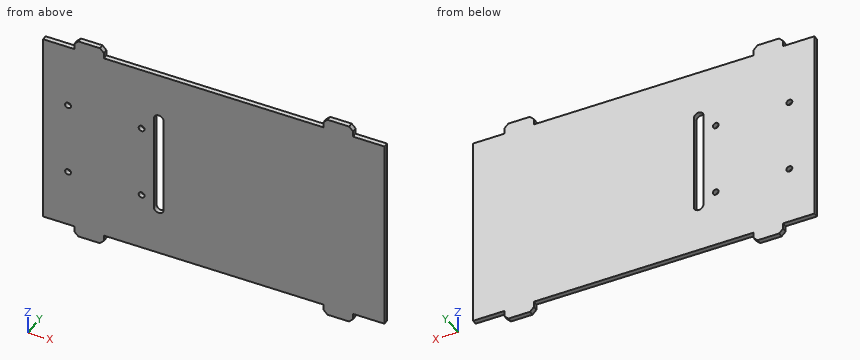
```python
from build123d import *

# Parameters (mm, degrees)
SKETCH1_W           = 174
SKETCH1_H           = 100
BOSS_EXTRUDE1_DEPTH = 2.5
SKETCH2_W           = 15
SKETCH2_H           = 2.5
BOSS_EXTRUDE2_DEPTH = 5
CHAMFER1_SIZE       = 2


with BuildPart() as part:
    # Sketch1 → Boss-Extrude1 (new body)
    with BuildSketch(Plane(origin=(0, 0, 0), x_dir=(1, 0, 0), z_dir=(0, 1, 0))):
        Rectangle(SKETCH1_W, SKETCH1_H)
        with BuildLine():
            Line((-25.5, 25), (-25.5, -25))
            ThreePointArc((-25.5, -25), (-28, -27.5), (-30.5, -25))
            Line((-30.5, -25), (-30.5, 25))
            ThreePointArc((-30.5, 25), (-28, 27.5), (-25.5, 25))
        make_face(mode=Mode.SUBTRACT)
        with BuildLine():
            ThreePointArc((-36.73295862, -15.609359563), (-38.23295862, -17.109359563), (-36.73295862, -18.609359563))
            ThreePointArc((-36.73295862, -18.609359563), (-35.23295862, -17.109359563), (-36.73295862, -15.609359563))
        make_face(mode=Mode.SUBTRACT)
        with BuildLine():
            ThreePointArc((-36.73295862, 18.890640437), (-35.23295862, 20.390640437), (-36.73295862, 21.890640437))
            ThreePointArc((-36.73295862, 21.890640437), (-38.23295862, 20.390640437), (-36.73295862, 18.890640437))
        make_face(mode=Mode.SUBTRACT)
        with BuildLine():
            ThreePointArc((-74.23295862, 21.890640437), (-75.73295862, 20.390640437), (-74.23295862, 18.890640437))
            ThreePointArc((-74.23295862, 18.890640437), (-72.73295862, 20.390640437), (-74.23295862, 21.890640437))
        make_face(mode=Mode.SUBTRACT)
        with BuildLine():
            ThreePointArc((-74.23295862, -15.609359563), (-75.73295862, -17.109359563), (-74.23295862, -18.609359563))
            ThreePointArc((-74.23295862, -18.609359563), (-72.73295862, -17.109359563), (-74.23295862, -15.609359563))
        make_face(mode=Mode.SUBTRACT)
    extrude(amount=BOSS_EXTRUDE1_DEPTH)

    # Sketch2 → Boss-Extrude2 (add)
    with BuildSketch(Plane.XY.offset(50)):
        with Locations((-63.5, 1.25)):
            Rectangle(SKETCH2_W, SKETCH2_H)
        with Locations((63.5, 1.25)):
            Rectangle(SKETCH2_W, SKETCH2_H)
    boss_extrude2 = extrude(amount=BOSS_EXTRUDE2_DEPTH)

    # Mirror1: Boss-Extrude2 across plane
    add(boss_extrude2.mirror(Plane.XY))

    # Chamfer1
    chamfer1_edges = [part.edges().sort_by_distance(p)[0] for p in [
        (-71, 1.25, 55),
        (-56, 1.25, 55),
        (56, 1.25, 55),
        (71, 1.25, 55),
        (-56, 1.25, -55),
        (-71, 1.25, -55),
        (71, 1.25, -55),
        (56, 1.25, -55),
    ]]
    chamfer(chamfer1_edges, length=CHAMFER1_SIZE)


solid = part.part
```
Source: CAD feature listing. Evaluate the final solid. Frame: model axes, mm. Round coordinates to 2 decimals unless told otherwise and drop trailing zeros. Loops run counter-clockwise (first coordinate to the right, second up) from the corner with the lowest first, then second, coordinate; pieces in that order, holes last. Notation, with made-up numbers: M -18.5,87 L -11.5,87 A8 ccw -11.5,95 Z; hole C -4.75,61 d9. An arc over 180 degrees is marked long. Use a Markdown table: item, result. Add a question column.
1. Cut plane C-C, the plane x = 17.5. Output: boundary loops of the cut face in (y, z), and give its area (3 significant figures).
2. Cut plane D-D, the plane y = 1.4. State how many separate pieces and enclosed holes the cut face has, and give its area (3 significant figures).
3. Cut plane A-A, the plane z = -1. Output: boundary loops of the cut face in (x, y).
4. Cut plane B-B, the plane x = -28. Output: boundary loops of the cut face in (y, z).
5. Ray query, line 1 along X through (y, z) = (2.25, 7); line 2 along Z through (x, y) = (-55.5, 0.8); line 3 along Z through (x, y) = (-26, 0.9). Return the intervals inside material, ascending. Write a range as [from, to].
6. Contact query for flat-ended pins moving along their axis: pin 1 (0.8 mm diameter, centred on x = 76.5, y = 1.5, fed in from -Z); pin 2 (0.8 mm diameter, centred on y = 1.5, z = -51.5, fed in from +X); pin 3 (0.8 mm diameter, centred on y = 1.5, z = -52, fed in from -X); pin 4 (2.5 mm diameter, centred on x = -74.23, z = 17.11, fed in from +Y). Output: stop coordinate, or through.
Solution:
| question | item | result |
|---|---|---|
| 1 | outline | M 0,-50 L 2.5,-50 L 2.5,50 L 0,50 Z |
| 1 | area | 250 mm2 |
| 2 | separate pieces | 1 |
| 2 | enclosed holes | 5 |
| 2 | area | 17,400 mm2 |
| 3 | outline | M -87,0 L -30.5,0 L -30.5,2.5 L -87,2.5 Z; M -25.5,0 L 87,0 L 87,2.5 L -25.5,2.5 Z |
| 4 | outline | M 0,-50 L 2.5,-50 L 2.5,-27.5 L 0,-27.5 Z; M 0,27.5 L 2.5,27.5 L 2.5,50 L 0,50 Z |
| 5 | line 1 | x = [-87, -30.5], [-25.5, 87] |
| 5 | line 2 | z = [-50, 50] |
| 5 | line 3 | z = [-50, -26.5], [26.5, 50] |
| 6 | pin 1 | stops at z = -50 |
| 6 | pin 2 | stops at x = 71 |
| 6 | pin 3 | stops at x = -71 |
| 6 | pin 4 | passes through |
